```python
from build123d import *

# Parameters (mm, degrees)
SKETCH1_W               = 70
SKETCH1_H               = 120
BOSS_EXTRUDE1_DEPTH     = 25
CUT_EXTRUDE1_DEPTH      = 61
CUT_EXTRUDE1_DEPTH_BACK = 61
BOSS_EXTRUDE6_DEPTH     = 25
BOSS_EXTRUDE7_DEPTH     = 21
RIB33_REACH             = 37
SKETCH10_WALL_W         = 128.291652
SKETCH10_WALL_H         = 10
FILLET1_R               = 3


with BuildPart() as part:
    # Sketch1 → Boss-Extrude1 (new body)
    with BuildSketch(Plane(origin=(0, 0, 0), x_dir=(1, 0, 0), z_dir=(0, 1, 0))):
        Rectangle(SKETCH1_W, SKETCH1_H)
    extrude(amount=BOSS_EXTRUDE1_DEPTH)

    # Sketch2 → Cut-Extrude1 (cut, two sides)
    with BuildSketch(Plane.XY) as cut_extrude1_sk:
        Polygon((-17, 0), (-24.505553, 13), (24.505553, 13), (17, 0), align=None)
    extrude(amount=CUT_EXTRUDE1_DEPTH, mode=Mode.SUBTRACT)
    extrude(cut_extrude1_sk.sketch, amount=-CUT_EXTRUDE1_DEPTH_BACK, mode=Mode.SUBTRACT)


with BuildPart() as body_2:
    # Sketch6 → Boss-Extrude6 (new, symmetric)
    with BuildSketch(Plane(origin=(0, 0, 0), x_dir=(0, 0, -1), z_dir=(1, 0, 0))):
        with BuildLine():
            ThreePointArc((11.5, 68), (-5.623611, 78.031201), (-6, 58.189292))
            ThreePointArc((-6, 58.189292), (0, 56.5), (6, 58.189292))
            ThreePointArc((6, 58.189292), (10.031201, 62.376389), (11.5, 68))
        make_face()
        with BuildLine():
            Line((-2.5, 75.071068), (-2.5, 77.571068))
            Line((-2.5, 77.571068), (2.5, 77.571068))
            Line((2.5, 77.571068), (2.5, 75.071068))
            ThreePointArc((2.5, 75.071068), (6.123724, 72.330127), (7.5, 68))
            ThreePointArc((7.5, 68), (-4.330127, 61.876276), (-2.5, 75.071068))
        make_face(mode=Mode.SUBTRACT)
    extrude(amount=BOSS_EXTRUDE6_DEPTH, both=True)


with BuildPart() as body_3:
    # Sketch6_3 → Boss-Extrude7 (new body)
    with BuildSketch(Plane(origin=(0, 0, 0), x_dir=(0, 0, -1), z_dir=(1, 0, 0))):
        with BuildLine():
            Line((-6, 58.189292), (-6, 25))
            Line((-6, 25), (6, 25))
            Line((6, 25), (6, 58.189292))
            ThreePointArc((6, 58.189292), (0, 56.5), (-6, 58.189292))
        make_face()
    extrude(amount=BOSS_EXTRUDE7_DEPTH)

    # Mirror4: body 3 across plane


with BuildPart() as body_3_1:
    add(body_3.part)
    add(body_3.part.mirror(Plane(origin=(0, 0, 0), x_dir=(0, 0, 1), z_dir=(1, 0, 0))))


with BuildPart() as body_2_1:
    add(body_2.part)

    # Combine2: union body 3, part
    add(body_3_1.part)
    add(part.part)

    # Sketch10 wall → Rib33 (add, up to next)
    with BuildSketch(Plane(origin=(0, 49.375, 24.032205), x_dir=(0, -0.866025, 0.5), z_dir=(0, -0.5, -0.866025)), mode=Mode.PRIVATE) as rib33_sk1:
        Rectangle(SKETCH10_WALL_W, SKETCH10_WALL_H)
    rib33_tool1 = extrude(rib33_sk1.sketch, amount=RIB33_REACH, mode=Mode.PRIVATE) - body_2_1.part
    rib33 = rib33_tool1.solids().sort_by_distance((0, 49.375, 24.032205))[0]
    add(rib33)

    # Mirror5: Rib33 across plane
    add(rib33.mirror(Plane.XY))

    # Fillet1
    fillet1_edges = [body_2_1.edges().sort_by_distance(p)[0] for p in [
        (5, 41.594646, -6),
        (5, 25, -22.052559),
        (-5, 41.594646, -6),
        (-5, 25, -22.052559),
        (0, 25, -38.105118),
        (13, 25, -6),
        (-21, 25, 0),
        (0, 25, -60),
        (-35, 25, 0),
        (21, 25, 0),
        (13, 25, 6),
        (0, 25, 60),
        (-35, 12.5, 60),
        (35, 25, 0),
        (35, 12.5, 60),
        (35, 12.5, -60),
        (-35, 12.5, -60),
        (-13, 25, 6),
        (5, 41.594646, 6),
        (5, 25, 22.052559),
        (-5, 25, 22.052559),
        (-5, 41.594646, 6),
        (0, 25, 38.105118),
        (-13, 25, -6),
    ]]
    fillet(fillet1_edges, radius=FILLET1_R)


solid = body_2_1.part
```
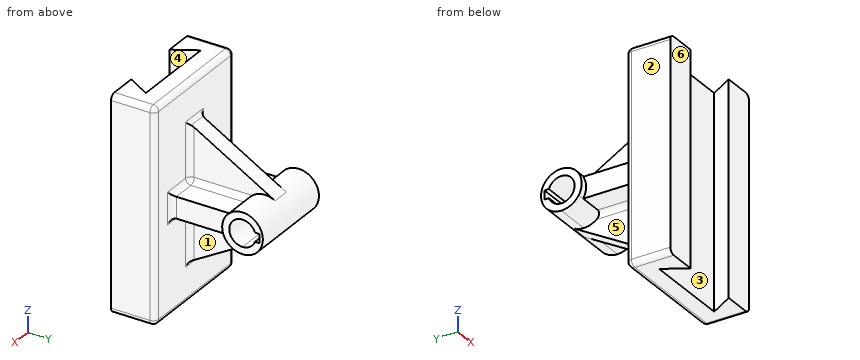
Can you work these out from the model? Positions are in its coordinate system, mm. Face numbers are marked on the shaded views. A direction names the side the tool comes from. Round coordinates to 2 decimals unless told otherwise and drop trailing zeros. Order: outer loops, then holes, each group sorted by start corner. A loop starts at its lowest first (then second) coordinate and runs counter-clockwise, first axis right, second up.
(1) If we section it at D-D (z = 25.5): Please give me the cut outline in (x, y), plus the area to 3 significant figures.
Results are:
outline: (-35, 0) - (-17, 0) - (-24.51, 13) - (24.51, 13) - (17, 0) - (35, 0) - (35, 22) arc R3 ccw to (32, 25) - (8, 25) arc R3 cw to (5, 28) - (5, 46.83) - (-5, 46.83) - (-5, 28) arc R3 cw to (-8, 25) - (-32, 25) arc R3 ccw to (-35, 22) - close
area: 1,430 mm2
(2) I'm going to push flat-ended pins straight in: pin 1 (6 mm diameter, centred on x = 4, y = 60, fed in from -Z); pin 2 (1 mm diameter, centred on y = 49, z = 18.5, fed in from +X); pin 3 (9.5 mm diameter, centred on y = 37.5, z = -1, fed in from -X); pin 4 (9 mm diameter, centred on y = 68, z = 0, fed in from -X). Where does each tip first touch, or does it pass through?
Results are:
pin 1: stops at z = -19.63
pin 2: stops at x = 5
pin 3: stops at x = -21
pin 4: passes through
(3) If we section it at B-B (x = -3.5): Please give me the cut outline in (y, z), plus the area to 3 significant figures.
Results are:
outline: (13, -60) - (22, -60) arc R3 ccw to (25, -57) - (25, -39.84) arc R3 cw to (26.5, -37.24) - (73.74, -9.96) arc R11.5 ccw to (73.74, 9.96) - (26.5, 37.24) arc R3 cw to (25, 39.84) - (25, 57) arc R3 ccw to (22, 60) - (13, 60) - close; hole (68, -7.5) arc R7.5 ccw to (75.07, -2.5) - (77.57, -2.5) - (77.57, 2.5) - (75.07, 2.5) arc R7.5 ccw (long way) to start
area: 3,670 mm2
(4) If we section it at A-A (z = 0): Please give me the cut outline in (x, y), plus the area to 3 significant figures.
Results are:
outline: (-35, 0) - (-17, 0) - (-24.51, 13) - (24.51, 13) - (17, 0) - (35, 0) - (35, 22) arc R3 ccw to (32, 25) - (24, 25) arc R3 cw to (21, 28) - (21, 56.5) - (25, 56.5) - (25, 60.5) - (-25, 60.5) - (-25, 56.5) - (-21, 56.5) - (-21, 28) arc R3 cw to (-24, 25) - (-32, 25) arc R3 ccw to (-35, 22) - close; (-25, 77.57) - (25, 77.57) - (25, 79.5) - (-25, 79.5) - close
area: 2,830 mm2
(5) If we section it at C-C (y = 70): Please give me the cut outline in (x, z), plus the area to 3 significant figures.
Results are:
outline: (-25, -11.32) - (-5, -11.32) - (-5, -12.12) - (5, -12.12) - (5, -11.32) - (25, -11.32) - (25, -7.23) - (-25, -7.23) - close; (-25, 7.23) - (25, 7.23) - (25, 11.32) - (5, 11.32) - (5, 12.12) - (-5, 12.12) - (-5, 11.32) - (-25, 11.32) - close
area: 426 mm2
(6) If I drill on L1, parallel to Z at x = 11, y = 68; L2, parallel to Y at x = -10, z = 0; L3, parallel to Z at x = 16, y = 35, over which ranges is the centre line in solid material (lowest first)?
Results are:
L1: z = -11.5 to -7.5, 7.5 to 11.5
L2: y = 13 to 60.5, 77.57 to 79.5
L3: z = -6 to 6
(7) We'd pull the mould along X, two halves only. Please class the marked faces 3, 4, 5 and 6: +X half, -X half, draft (parallel to the pull), parting line (faces both ways), or undercut.
Results are:
face 3: undercut
face 4: undercut
face 5: -X half
face 6: draft
(8) On a 3-axis mill with a long thin cutter (end or side, diameter ignored), from which of +Z, -Z, +X, -X, +Y, -Y can I reach the whole of each face in a straight line? I mean the marked faces 1 and 2. Say none if no direction works.
Results are:
face 1: -Z, +X
face 2: +Z, -Z, -X, +Y, -Y
